The listing builds one solid part. Answer for the finished solid, in the listing's coordinates (mm). A direction names the side the tool comes from. Round coordinates to 2 decimals unless told otherwise and drop trailing zeros. Write each loop counter-clockwise with the first axis right and the second up, starting at its lowest first coordinate (ties: lowest second). Pieces come first, ordered by that corner, then holes. Notation, with made-up numbers: (71, 79) - (115, 79) arc R26 cw to (115, 118) - close; hole circle Ø11 at (58, 59). An arc over 180 degrees is marked (long way). Return JSON: item names as keys, results as strings. Group by question number.
Autodesk Inventor part; units mm, degrees
ref_plane "YZ Plane" through (0, 0, 0) normal (1, 0, 0) x (0, 1, 0)
ref_plane "XZ Plane" through (0, 0, 0) normal (0, 1, 0) x (-1, 0, 0)
ref_plane "XY Plane" through (0, 0, 0) normal (0, 0, 1) x (1, 0, 0)
sketch "Эскиз1" plane through (0, 0, 0) normal (0, 0, 1) x (1, 0, 0)
  line L0 (0, 0) -> (-282.435, 0)
  line L1 (0, 0) -> (0, 30)
  line L2 (-10, 40) -> (-30, 40)
  line L3 (-30, 40) -> (-30, 30)
  line L4 (-30, 30) -> (-230, 30)
  line L5 (-230, 30) -> (-230, 0)
  arc A0 (0, 30) -> (-10, 40) centre (-10, 30) ccw
  point P0 (0, 40)
  dimension "d0" = 230
  dimension "d1" = 80
  dimension "d2" = 60
  dimension "d3" = 30
  dimension "d4" = 10
revolve "Вращение1" add sketch "Эскиз1" angle 360 about axis through (0, 0, 0) along (-1, 0, 0)
sketch "Эскиз2" plane through (0, 0, 0) normal (0, 1, 0) x (-1, 0, 0)
  line L0 (230, 30) -> (230, -30)
  line L1 (30, 30) -> (30, -30)
  circle A0 centre (210, 0) radius 6
  point P0 (0, 0)
  point P1 (230, 0)
  dimension "d6" = 12
  dimension "d7" = 20
extrude "Выдавливание1" cut sketch "Эскиз2" against normal through all both and the other way through all
properties part number "Lift.03.00.00.03"
(1) For faces 4 (the flat face through (-30, 6, -30)), 5 (the flat face through (-230, 0, 0)), determine the directions among +Z, -Z, +X, -X, +Y, -Y from which every point of the face is accessible in a straight line to the end or side of a thin tool.
(2) Consider line 1 (Z direction, x = -210, y = -1); line 2 (Y direction, x = -138, z = -1); line 3 (Z direction, x = -210, y = 14.5). Determine where each line is inside the solid, lowest interval first.
(3) Find section B-B (z = 0). Write down the section's boundary in (x, y), plus the area to 3 significant figures.
(4) Find section A-A (y = 0). Write down the section's boundary in (x, z).
(5) Find section C-C (x = -16). Write down the section's boundary in (y, z), plus the area to 3 significant figures.
(6) Flat-ended cylindrical pins translate along their axes: pin 1 (5 mm diameter, centred on x = -89, z = 6.5, fed in from -Y); pin 2 (4 mm diameter, centred on x = -192.5, z = 21, fed in from +Y); pin 3 (3 mm diameter, centred on x = -70.5, z = 21.5, fed in from +Y). Find the tip coordinate at first contact, or state that the pin passes through.
(7) Find section D-D (x = -210). Write down the section's boundary in (y, z), plus the area to 3 significant figures.
(8) Determine the mould class of faces 1 (the flat face through (0, 0, 0)), 2 (the cylindrical face through (-205.24, 0.42, -3.65)), 3 (the cylindrical face through (-20.14, -8.67, 39.05)) for opening direction Z: +Z half, -Z half, draft (parallel to the pull), parting line (faces both ways), or undercut.
Check sheet entries:
{
 "1": {"face 4": "-X", "face 5": "+Z, -Z, -X, +Y, -Y"},
 "2": {"line 1": "z = -29.98 to -6, 6 to 29.98", "line 2": "y = -29.98 to 29.98", "line 3": "z = -26.26 to -6, 6 to 26.26"},
 "3": {"outline": "(-230, -30) - (-216, -30) - (-216, 30) - (-230, 30) - close; (-204, -30) - (-30, -30) - (-30, -40) - (-10, -40) arc R10 ccw to (0, -30) - (0, 30) arc R10 ccw to (-10, 40) - (-30, 40) - (-30, 30) - (-204, 30) - close", "area": "13,600 mm^2"},
 "4": {"outline": "(-230, -30) - (-30, -30) - (-30, -40) - (-10, -40) arc R10 ccw to (0, -30) - (0, 30) arc R10 ccw to (-10, 40) - (-30, 40) - (-30, 30) - (-230, 30) - close; hole circle Ø12 at (-210, 0)"},
 "5": {"outline": "circle Ø80 at (0, 0)", "area": "5,030 mm^2"},
 "6": {"pin 1": "stops at y = -29.73", "pin 2": "stops at y = 23.22", "pin 3": "stops at y = 22.36"},
 "7": {"outline": "(-29.39, -6) arc R30 ccw to (29.39, -6) - close; (-29.39, 6) - (29.39, 6) arc R30 ccw to start", "area": "2,110 mm^2"},
 "8": {"face 1": "draft", "face 2": "undercut", "face 3": "parting line"}
}
